Geometry check sheet. Reference: drawing and pictorial views, mm from the part's lowest x, y, z. A direction names the side the tool comes from. Give positions to 0.01 mm unless a question says otherwise; leave off trailing zeros. Order: outer loops, then holes, each group sorted by start corner. A loop starts at its lowest first (then second) coordinate and runs counter-clockwise, first axis right, second up. Notation, with made-up numbers: (80, -23) - (110, -23) arc R26 cw to (110, 10) - close; hole circle Ø2 at (-33, 53). An arc over 180 degrees is marked (long way). Answer in a Markdown table with one row per item.
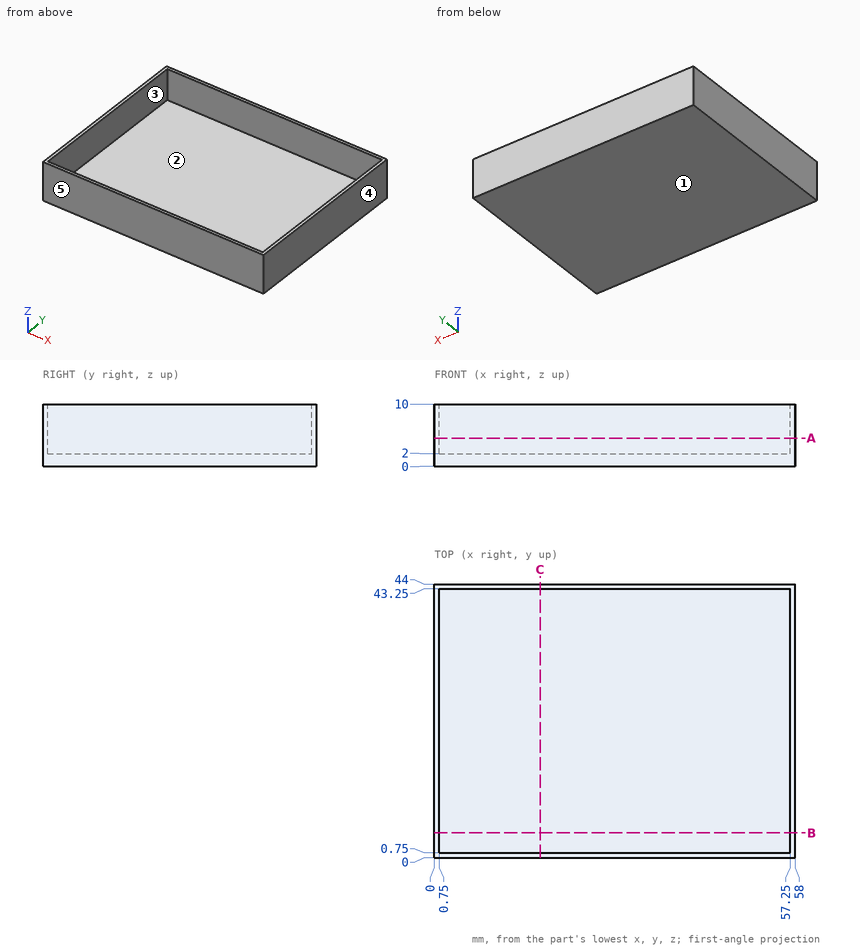
(1) Cross-section at C-C, the plane x = 17. Record the cut outline in (y, z).
Geometry says:
| item | result |
|---|---|
| outline | (0, 0) - (44, 0) - (44, 10) - (43.25, 10) - (43.25, 2) - (0.75, 2) - (0.75, 10) - (0, 10) - close |
(2) Cross-section at A-A, the plane z = 4.5. Record the cut outline in (x, y).
Geometry says:
| item | result |
|---|---|
| outline | (0, 0) - (58, 0) - (58, 44) - (0, 44) - close; hole (0.75, 0.75) - (57.25, 0.75) - (57.25, 43.25) - (0.75, 43.25) - close |
(3) Cross-section at B-B, the plane y = 4. Record the cut outline in (x, z), then the cut area to 3 significant figures.
Geometry says:
| item | result |
|---|---|
| outline | (0, 0) - (58, 0) - (58, 10) - (57.25, 10) - (57.25, 2) - (0.75, 2) - (0.75, 10) - (0, 10) - close |
| area | 128 mm² |
(4) Mould release check, pull along X, two halves, no side actions. Record for the marked faces 3, 4 and 5: pulls with the +X half, pulls with the -X half, needs draft (parallel to the pull), parting line crosses it, or undercut.
Geometry says:
| item | result |
|---|---|
| face 3 | undercut |
| face 4 | pulls with the +X half |
| face 5 | needs draft |
(5) Access from +Z, -Z, +X, -X, +Y, -Y to the whole of each face (thin tool, end or side, straight path). Record for the marked faces 1 and 2.
Geometry says:
| item | result |
|---|---|
| face 1 | -Z, +X, -X, +Y, -Y |
| face 2 | +Z |
(6) Thickness scan on L1, parallel to Y at x = 24, z = 7; L2, parallel to X at y = 7.5, z = 7; L3, parallel to Z at x = 12, y = 4.5. Record the ranges inside material, lowest first.
Geometry says:
| item | result |
|---|---|
| L1 | 0 to 0.75, 43.25 to 44 |
| L2 | 0 to 0.75, 57.25 to 58 |
| L3 | 0 to 2 |
